```python
from build123d import *

# Parameters (mm, degrees)
F1_DEPTH      = 10
F1_DEPTH_BACK = 10
F3_D          = 4
F5_D          = 4
F5_DEPTH      = 18.2076214093
F7_D          = 8
F8_R          = 3
F9_R          = 5
F11_D         = 4


with BuildPart() as f1:
    # F0 (on Front) → F1 (new body, two sides)
    with BuildSketch(Plane.XZ) as f1_sk:
        Polygon((-40.2948366535, -6.0925860852), (-36.1803398875, -11.7557050458), (-20, 0), (15, 0), (26.7557050458, -16.1803398875), (32.4188240065, -12.0658431215), (18.5666781465, 7), (-22.2744378736, 7), align=None)
    extrude(amount=F1_DEPTH)
    extrude(f1_sk.sketch, amount=-F1_DEPTH_BACK)

    # F3 (through all)
    with Locations(Plane(origin=(-6.9098300563, 0, 9.510565163), x_dir=(0.8090169944, 0, 0.5877852523), z_dir=(0.5877852523, 0, -0.8090169944))):
        with Locations((0, -37.8532769899), (0, -24.0082326065), (-30.1803398875, 0), (-21.1803398875, 0)):
            Hole(F3_D / 2)

    # F5 (through all, one way)
    with BuildSketch(Plane(origin=(9.8176274578, 0, 7.1329238722), x_dir=(0, -1, 0), z_dir=(-0.8090169944, 0, -0.5877852523))):
        with Locations((16.0583042515, 0), (-6.1736582538, 0)):
            Circle(F5_D / 2)
    extrude(amount=-F5_DEPTH, mode=Mode.SUBTRACT)

    # F7 (through all)
    with Locations(Plane(origin=(0, 0, 0), x_dir=(1, 0, 0), z_dir=(0, 0, -1))):
        with Locations((0, 0)):
            Hole(F7_D / 2)

    # F8
    f8_edges = [f1.edges().sort_by_distance(p)[0] for p in [
        (-36.18034, 0, -11.755705),
        (26.755705, 0, -16.18034),
    ]]
    fillet(f8_edges, radius=F8_R)

    # F9
    f9_edges = [f1.edges().sort_by_distance(p)[0] for p in [
        (-20, 0, 0),
        (15, 0, 0),
    ]]
    fillet(f9_edges, radius=F9_R)

    # F11 (through all)
    with Locations(Plane(origin=(9.8176274578, 0, 7.1329238722), x_dir=(0, -1, 0), z_dir=(-0.8090169944, 0, -0.5877852523))):
        with Locations((0, -15.1145784184), (0, -22.5539375097)):
            Hole(F11_D / 2)


solid = f1.part
```
Could you check a few things on this model? Use its own coordinates, in mm. A direction names the side the tool comes from. Give positions to 0.01 mm unless a question says otherwise; leave off trailing zeros. Loops run counter-clockwise (first coordinate to the right, second up) from the corner with the lowest first, then second, coordinate; pieces in that order, holes last. Notation, with made-up numbers: (31, 63) - (71, 63) arc R20 cw to (71, 100) - close; hole circle Ø5 at (49.25, 89.25). An arc over 180 degrees is marked (long way). Answer in a Markdown table with one row per item. Add a question column.
Q1. If we section it at A-A (x = 0): List the corners of the cut face in (y, z) for me.
Q2. If we section it at D-D (y = 0): State how many separate pieces and enclosed holes the cut face has, plus the area to 3 significant figures.
Q3. If we section it at C-C (y = -6.75): List the corners of the cut face in (x, z) for me, plus the area to 3 significant figures.
Q4. If we section it at B-B (y = -3.25): List the corners of the cut face in (x, z) for me.
Q5. Which directions (+Z, -Z, +X, -X, +Y, -Y) give clear straight access to the entire face, cutting with the end or side of a thin tool? Please do faces 4 (the face through (11.8, 6.2, 6.1)), 5 (the face through (25.59, 2.08, -2.67)), 6 (the face through (14.69, -0.14, -0.53)).
Q6. For pin 1 (1 mm diameter, centred on y = -2, z = -1, fed in from +X); pin 2 (8 mm diameter, centred on y = 6, z = -3.5, fed in from -X); pin 3 (12 mm diameter, centred on x = -19, y = -6.5, fed in from -Z), each with a flat end and sliding along its axis, tell me the tip position at first contact or that it passes through.
Q7. We'd pull the mould along Z, two halves only. Please class faces 1 (the face through (0.867, 3.905, 3.549)), 2 (the face through (10.33, 6.2, 6.43)), 3 (the face through (-24.515, -0.088, 1.107)): +Z half, -Z half, draft (parallel to the pull), parting line (faces both ways), or undercut.
Q8. Please list where these lines run through material, in increasing order: L1, parallel to Y at x = 0, z = 4.5; L2, parallel to Z at x = -16.5, y = -1.75; L3, parallel to X at y = 6.25, z = -6. Write a range as from..to.
The answers:
| question | item | result |
|---|---|---|
| 1 | outline | (-10, 0) - (-4, 0) - (-4, 7) - (-10, 7) - close; (4, 0) - (10, 0) - (10, 7) - (4, 7) - close |
| 2 | separate pieces | 6 |
| 2 | enclosed holes | 0 |
| 2 | area | 395 mm^2 |
| 3 | outline | (-40.29, -6.09) - (-37.94, -9.33) arc R3 ccw to (-33.75, -9.99) - (-21.31, -0.95) arc R5 cw to (-18.38, 0) - (12.45, 0) arc R5 cw to (16.5, -2.06) - (24.99, -13.75) arc R3 ccw to (29.18, -14.42) - (32.42, -12.07) - (18.57, 7) - (-22.27, 7) - close |
| 3 | area | 563 mm^2 |
| 4 | outline | (-40.29, -6.09) - (-37.94, -9.33) arc R3 ccw to (-33.75, -9.99) - (-21.31, -0.95) arc R5 cw to (-18.38, 0) - (-2.33, 0) - (-2.33, 7) - (-22.27, 7) - close; (2.33, 0) - (12.45, 0) arc R5 cw to (16.5, -2.06) - (24.99, -13.75) arc R3 ccw to (29.18, -14.42) - (32.42, -12.07) - (18.57, 7) - (2.33, 7) - close |
| 5 | face 4 | +Z |
| 5 | face 5 | +Z, +X, +Y, -Y |
| 5 | face 6 | -Z, +Y, -Y |
| 6 | pin 1 | stops at x = 24.74 |
| 6 | pin 2 | stops at x = -40.29 |
| 6 | pin 3 | stops at z = -3.63 |
| 7 | face 1 | draft |
| 7 | face 2 | +Z half |
| 7 | face 3 | undercut |
| 8 | L1 | y = -10..-4, 4..10 |
| 8 | L2 | z = 0..7 |
| 8 | L3 | x = -40.17..-28.26, 19.36..28.01 |
